Could you check a few things on this model? Use its own coordinates, in mm. Give positions to 0.01 mm unless a question says otherwise; leave off trailing zeros. Loops run counter-clockwise (first coordinate to the right, second up) from the corner with the lowest first, then second, coordinate; pieces in that order, holes last. Notation, with made-up numbers: (1.25, 88.25) - (23.25, 88.25) arc R17 cw to (23.25, 98.25) - close; hole circle Ø2 at (-21.5, 74). An arc over 180 degrees is marked (long way). Use CSV: the item, a comma, the result in double quotes.
from build123d import *

# Parameters (mm, degrees)
F1_DEPTH = 762


# Not quite as in the source:
# - ends of sketch curves that miss each other by under 0.0002 mm in the source are joined


with BuildPart() as f1:
    # F0 (on Top) → F1 (new body)
    with BuildSketch(Plane.XY):
        with BuildLine():
            ThreePointArc((488.8742323068, 15.2944921486), (487.5203307918, 14.9025505993), (487.1193724988, 16.2538092487))
            ThreePointArc((487.1193724988, 16.2538092487), (481.824523523, 18.9352573397), (476.4205037428, 21.389266255))
            ThreePointArc((476.4205037428, 21.389266255), (475.1125647356, 20.8581030883), (474.5767217389, 22.1641318166))
            ThreePointArc((474.5767217389, 22.1641318166), (463.1842997703, 26.2876905948), (451.4772940324, 29.4081123545))
            ThreePointArc((451.4772940324, 29.4081123545), (450.276485478, 28.6452994006), (449.5280311535, 29.8551096795))
            ThreePointArc((449.5280311535, 29.8551096795), (438.0355044136, 32.4749833354), (426.4826400862, 34.8144778691))
            ThreePointArc((426.4826400862, 34.8144778691), (425.3154916622, 34.0171690515), (424.5169792351, 35.1834943482))
            ThreePointArc((424.5169792351, 35.1834943482), (413.0262686458, 37.1733622263), (401.4909912337, 38.8860732489))
            ThreePointArc((401.4909912337, 38.8860732489), (400.3671427029, 38.0288648232), (399.5087220344, 39.1517876884))
            ThreePointArc((399.5087220344, 39.1517876884), (375.5310617416, 42.0658475749), (351.4961188511, 44.4619816239))
            ThreePointArc((351.4961188511, 44.4619816239), (350.4124269023, 43.5538419038), (349.5038028578, 44.6371278018))
            ThreePointArc((349.5038028578, 44.6371278018), (325.5182950967, 46.4647415416), (301.4990594281, 47.7766380455))
            ThreePointArc((301.4990594281, 47.7766380455), (300.4634214455, 46.8206692193), (299.5004439239, 47.8497934687))
            ThreePointArc((299.5004439239, 47.8497934687), (250.4170586651, 48.9784061279), (201.3229831968, 49.4519342839))
            ThreePointArc((201.3229831968, 49.4519342839), (200.4972514489, 49.0200037773), (199.6739065342, 49.4564668725))
            ThreePointArc((199.6739065342, 49.4564668725), (150.5832624149, 49.2528772685), (101.4997048201, 48.3942955287))
            ThreePointArc((101.4997048201, 48.3942955287), (101.4999262023, 48.3821486609), (101.5, 48.37))
            ThreePointArc((101.5, 48.37), (100.5122846343, 47.370075459), (99.5003018245, 48.3454325854))
            ThreePointArc((99.5003018245, 48.3454325854), (50.4236366017, 46.8049664772), (1.3719002627, 44.6096835018))
            ThreePointArc((1.3719002627, 44.6096835018), (1.4674451568, 44.3730807552), (1.5, 44.12))
            ThreePointArc((1.5, 44.12), (0.297194356, 43.1407809894), (-0.4177397415, 44.5171822841))
            ThreePointArc((-0.4177397415, 44.5171822841), (-49.4818219256, 41.6405010198), (-98.503098248, 38.1086568293))
            ThreePointArc((-98.503098248, 38.1086568293), (-98.5007748622, 38.0693589124), (-98.5, 38.03))
            ThreePointArc((-98.5, 38.03), (-99.4653855857, 37.0305992584), (-100.4976036846, 37.9608126573))
            ThreePointArc((-100.4976036846, 37.9608126573), (-149.5105569813, 34.4207797542), (-198.5029069122, 30.606193006))
            ThreePointArc((-198.5029069122, 30.606193006), (-198.5007269923, 30.568124219), (-198.5, 30.53))
            ThreePointArc((-198.5, 30.53), (-199.4575267193, 29.5309023969), (-200.4963920408, 30.445130094))
            ThreePointArc((-200.4963920408, 30.445130094), (-249.5122047164, 26.3409146536), (-298.5042296621, 21.9618772772))
            ThreePointArc((-298.5042296621, 21.9618772772), (-298.5010579752, 21.915987292), (-298.5, 21.87))
            ThreePointArc((-298.5, 21.87), (-299.4539559536, 20.8710605895), (-300.4957598916, 21.7780095749))
            ThreePointArc((-300.4957598916, 21.7780095749), (-349.5135367847, 17.1080068146), (-398.5043233752, 12.1628873449))
            ThreePointArc((-398.5043233752, 12.1628873449), (-398.5010814285, 12.1164939523), (-398.5, 12.07))
            ThreePointArc((-398.5, 12.07), (-399.443021479, 11.0716245956), (-400.4935068963, 11.9562280921))
            ThreePointArc((-400.4935068963, 11.9562280921), (-424.5032598568, 9.4256444152), (-448.5059560316, 6.8289797637))
            ThreePointArc((-448.5059560316, 6.8289797637), (-448.5014901181, 6.7745711994), (-448.5, 6.72))
            ThreePointArc((-448.5, 6.72), (-449.4453720697, 5.7214932202), (-450.4940315785, 6.6109072825))
            ThreePointArc((-450.4940315785, 6.6109072825), (-474.5067314104, 3.9406998666), (-498.5119845054, 1.2043547292))
            ThreePointArc((-498.5119845054, 1.2043547292), (-498.5030006282, 1.1274096421), (-498.5, 1.05))
            ThreePointArc((-498.5, 1.05), (-499.2142366184, 0.0916997914), (-500.3366785795, 0.5023057837))
            ThreePointArc((-500.3366785795, 0.5023057837), (-500.458136, 0), (-500.3366785795, -0.5023057837))
            ThreePointArc((-500.3366785795, -0.5023057837), (-499.2142366184, -0.0916997914), (-498.5, -1.05))
            ThreePointArc((-498.5, -1.05), (-498.5030005898, -1.1274091465), (-498.5119843519, -1.2043537469))
            ThreePointArc((-498.5119843519, -1.2043537469), (-474.5067312795, -3.9406988813), (-450.49403147, -6.6109062944))
            ThreePointArc((-450.49403147, -6.6109062944), (-449.4453715735, -5.7214932474), (-448.5, -6.72))
            ThreePointArc((-448.5, -6.72), (-448.501490091, -6.7745707031), (-448.5059559233, -6.8289787756))
            ThreePointArc((-448.5059559233, -6.8289787756), (-424.5032597461, -9.425643427), (-400.4935067831, -11.9562271039))
            ThreePointArc((-400.4935067831, -11.9562271039), (-399.4430209825, -11.0716246239), (-398.5, -12.07))
            ThreePointArc((-398.5, -12.07), (-398.5010814054, -12.1164934555), (-398.5043232828, -12.1628863545))
            ThreePointArc((-398.5043232828, -12.1628863545), (-349.5135366927, -17.1080058236), (-300.4957598, -21.7780085834))
            ThreePointArc((-300.4957598, -21.7780085834), (-299.4539554563, -20.8710606125), (-298.5, -21.87))
            ThreePointArc((-298.5, -21.87), (-298.5010579523, -21.9159867947), (-298.5042295706, -21.9618762856))
            ThreePointArc((-298.5042295706, -21.9618762856), (-249.5122046283, -26.3409136613), (-200.4963919562, -30.4451291009))
            ThreePointArc((-200.4963919562, -30.4451291009), (-199.4575262213, -29.5309024181), (-198.5, -30.53))
            ThreePointArc((-198.5, -30.53), (-198.5007269733, -30.568123721), (-198.5029068362, -30.6061920122))
            ThreePointArc((-198.5029068362, -30.6061920122), (-149.5105569088, -34.4207787596), (-100.4976036156, -37.9608116621))
            ThreePointArc((-100.4976036156, -37.9608116621), (-99.4653850872, -37.0305992757), (-98.5, -38.03))
            ThreePointArc((-98.5, -38.03), (-98.5007748622, -38.0693589124), (-98.503098248, -38.1086568293))
            ThreePointArc((-98.503098248, -38.1086568293), (-49.4818219256, -41.6405010198), (-0.4177397415, -44.5171822841))
            ThreePointArc((-0.4177397415, -44.5171822841), (0.297194356, -43.1407809894), (1.5, -44.12))
            ThreePointArc((1.5, -44.12), (1.4674451568, -44.3730807552), (1.3719002627, -44.6096835018))
            ThreePointArc((1.3719002627, -44.6096835018), (50.4236366017, -46.8049664772), (99.5003018245, -48.3454325854))
            ThreePointArc((99.5003018245, -48.3454325854), (100.5122846343, -47.370075459), (101.5, -48.37))
            ThreePointArc((101.5, -48.37), (101.4999262023, -48.3821486609), (101.4997048201, -48.3942955287))
            ThreePointArc((101.4997048201, -48.3942955287), (150.5832624149, -49.2528772685), (199.6739065342, -49.4564668725))
            ThreePointArc((199.6739065342, -49.4564668725), (200.4972514489, -49.0200037773), (201.3229831968, -49.4519342839))
            ThreePointArc((201.3229831968, -49.4519342839), (250.4170586651, -48.9784061279), (299.5004439239, -47.8497934687))
            ThreePointArc((299.5004439239, -47.8497934687), (300.4634214455, -46.8206692193), (301.4990594281, -47.7766380455))
            ThreePointArc((301.4990594281, -47.7766380455), (325.5182950967, -46.4647415416), (349.5038028578, -44.6371278018))
            ThreePointArc((349.5038028578, -44.6371278018), (350.4124269023, -43.5538419038), (351.4961188511, -44.4619816239))
            ThreePointArc((351.4961188511, -44.4619816239), (375.5310617416, -42.0658475749), (399.5087220344, -39.1517876884))
            ThreePointArc((399.5087220344, -39.1517876884), (400.3671422118, -38.0288648891), (401.490991101, -38.886072267))
            ThreePointArc((401.490991101, -38.886072267), (413.0262684891, -37.1733612515), (424.5169790547, -35.1834933817))
            ThreePointArc((424.5169790547, -35.1834933817), (425.3154916626, -34.0171690514), (426.4826399039, -34.8144769037))
            ThreePointArc((426.4826399039, -34.8144769037), (438.035504208, -32.4749823797), (449.5280309249, -29.8551087345))
            ThreePointArc((449.5280309249, -29.8551087345), (450.2764859518, -28.645299292), (451.4772940324, -29.4081123545))
            ThreePointArc((451.4772940324, -29.4081123545), (463.1842997703, -26.2876905948), (474.5767217389, -22.1641318166))
            ThreePointArc((474.5767217389, -22.1641318166), (475.1125647356, -20.8581030883), (476.4205037428, -21.389266255))
            ThreePointArc((476.4205037428, -21.389266255), (481.824523523, -18.9352573397), (487.1193724988, -16.2538092487))
            ThreePointArc((487.1193724988, -16.2538092487), (487.5203307918, -14.9025505993), (488.8742323068, -15.2944921486))
            ThreePointArc((488.8742323068, -15.2944921486), (496.019452289, -9.0885932824), (500.3796021729, -0.6888050517))
            ThreePointArc((500.3796021729, -0.6888050517), (500.4696732905, -0.3496239971), (500.499999, 0))
            ThreePointArc((500.499999, 0), (500.4696732095, 0.3496244605), (500.379601649, 0.6888058734))
            ThreePointArc((500.379601649, 0.6888058734), (496.0194519925, 9.0885936587), (488.8742323068, 15.2944921486))
        make_face()
    extrude(amount=-F1_DEPTH)


solid = f1.part
1) Suppose I cut it at A-A (x = -377). Please give me the cut outline in (y, z), plus the area to 3 significant figures.
Answer below:
outline,"(-14.37, -762) - (14.37, -762) - (14.37, 0) - (-14.37, 0) - close"
area,"21,900 mm2"
2) I'm going to push flat-ended pins straight in: P1, Ø5, axis at y = 12, z = -371.5, coming from the +X side; P2, Ø4, axis at x = -363, z = -293.5, coming from the -Y side; P3, Ø3, axis at y = -10, z = -471, coming from the +X side. Where does each tip first touch, or does it pass through?
Answer below:
P1,"stops at x = 495.69"
P2,"stops at y = -15.97"
P3,"stops at x = 496.47"
3) I need wall thicknesses on line 1 along Y through (x, z) = (-223, -561); line 2 along Y through (x, z) = (0.5, -394.5); line 3 along X through (y, z) = (-1, -670.5). Which ranges of each line are inside material? Lowest first, please.
Answer below:
line 1,"y = -28.6 to 28.6"
line 2,"y = -43.12 to 43.12"
line 3,"x = -498.5 to 500.28"
4) Suppose I cut it at B-B (x = 42). Please give me the cut outline in (y, z), plus the area to 3 significant figures.
Answer below:
outline,"(-46.47, -762) - (46.47, -762) - (46.47, 0) - (-46.47, 0) - close"
area,"70,800 mm2"
